```python
from build123d import *

# Parameters (mm, degrees)
SKETCH2_R           = 4.5
BOSS_EXTRUDE1_DEPTH = 17
SKETCH3_R           = 9
BOSS_EXTRUDE2_DEPTH = 18
SKETCH4_R           = 8
BOSS_EXTRUDE3_DEPTH = 29
SKETCH5_R           = 9
BOSS_EXTRUDE4_DEPTH = 15
SKETCH6_R           = 3
BOSS_EXTRUDE5_DEPTH = 20
BOSS_EXTRUDE6_DEPTH = 4
SKETCH17_R          = 3
BOSS_EXTRUDE7_DEPTH = 5
SKETCH18_R          = 9
BOSS_EXTRUDE8_DEPTH = 16
CUT_EXTRUDE1_DEPTH  = 3


with BuildPart() as part:
    # Sketch2 → Boss-Extrude1 (new body)
    with BuildSketch(Plane.YZ):
        Circle(SKETCH2_R)
    extrude(amount=BOSS_EXTRUDE1_DEPTH)

    # Sketch3 → Boss-Extrude2 (add)
    with BuildSketch(Plane(origin=(0, 0, 0), x_dir=(0, -1, 0), z_dir=(-1, 0, 0))):
        Circle(SKETCH3_R)
    extrude(amount=BOSS_EXTRUDE2_DEPTH)

    # Sketch4 → Boss-Extrude3 (add)
    with BuildSketch(Plane(origin=(-18, 0, 0), x_dir=(0, -1, 0), z_dir=(-1, 0, 0))):
        Circle(SKETCH4_R)
    extrude(amount=BOSS_EXTRUDE3_DEPTH)

    # Sketch5 → Boss-Extrude4 (add)
    with BuildSketch(Plane(origin=(-47, 0, 0), x_dir=(0, -1, 0), z_dir=(-1, 0, 0))):
        with Locations((0, -0.197923741)):
            Circle(SKETCH5_R)
    extrude(amount=BOSS_EXTRUDE4_DEPTH)

    # Sketch6 → Boss-Extrude5 (add)
    with BuildSketch(Plane(origin=(-62, 0, 0), x_dir=(0, -1, 0), z_dir=(-1, 0, 0))):
        Circle(SKETCH6_R)
    extrude(amount=BOSS_EXTRUDE5_DEPTH)

    # Sketch16 → Boss-Extrude6 (add, symmetric)
    with BuildSketch(Plane(origin=(0, 0, 0), x_dir=(0, 1, 0), z_dir=(0, 0, 1))):
        with BuildLine():
            Line((0, 62), (-20, 62))
            ThreePointArc((-20, 62), (-34.142135624, 67.857864376), (-40, 82))
            Line((-40, 82), (-40, 102))
            ThreePointArc((-40, 102), (-34.142135624, 116.142135624), (-20, 122))
            Line((-20, 122), (0, 122))
            Line((0, 122), (0, 138))
            Line((0, 138), (-12, 138))
            Line((-12, 138), (-28.922313782, 140.983860496))
            ThreePointArc((-28.922313782, 140.983860496), (-57.497566339, 133.327144649), (-70, 106.51558914))
            Line((-70, 106.51558914), (-70, 82))
            ThreePointArc((-70, 82), (-59.748737342, 57.251262658), (-35, 47))
            Line((-35, 47), (0, 47))
            Line((0, 47), (0, 62))
        make_face()
    extrude(amount=BOSS_EXTRUDE6_DEPTH, both=True)



with BuildPart() as body_2:
    # Sketch17 → Boss-Extrude7 (new body)
    with BuildSketch(Plane.ZY.offset(117)):
        Circle(SKETCH17_R)
    extrude(amount=BOSS_EXTRUDE7_DEPTH)


with BuildPart() as part_1:
    add(part.part)

    add(body_2.part)  # Boss-Extrude8 merges body 2
    # Sketch18 → Boss-Extrude8 (add)
    with BuildSketch(Plane(origin=(-122, 0, 0), x_dir=(0, -1, 0), z_dir=(-1, 0, 0))):
        Circle(SKETCH18_R)
    extrude(amount=BOSS_EXTRUDE8_DEPTH)

    # Sketch21 → Cut-Extrude1 (cut)
    with BuildSketch(Plane.XY.offset(4)):
        with BuildLine():
            Line((-106.51558914, -65), (-82, -65))
            ThreePointArc((-82, -65), (-60.786796564, -56.213203436), (-52, -35))
            Line((-52, -35), (-52, -24.70089464))
            ThreePointArc((-52, -24.70089464), (-54.470885592, -22.009811643), (-57.362613993, -24.24254767))
            ThreePointArc((-57.362613993, -24.24254767), (-65.891984786, -39.11888715), (-82, -45))
            Line((-82, -45), (-102, -45))
            ThreePointArc((-102, -45), (-117.587304364, -39.545739757), (-126.373231569, -25.562875413))
            ThreePointArc((-126.373231569, -25.562875413), (-130.955140822, -22.001423997), (-135.353853676, -25.786810875))
            Line((-135.353853676, -25.786810875), (-136.059821731, -29.79055467))
            ThreePointArc((-136.059821731, -29.79055467), (-129.496922434, -54.283628291), (-106.51558914, -65))
        make_face()
    cut_extrude1 = extrude(amount=-CUT_EXTRUDE1_DEPTH, mode=Mode.SUBTRACT)

    # Mirror1: Cut-Extrude1 across plane
    add(cut_extrude1.mirror(Plane.XY), mode=Mode.SUBTRACT)


solid = part_1.part
```
Input: part model. Units: mm. Frame: model coordinates. A direction names the side the tool comes from. Give positions to 0.01 mm unless a question says otherwise; leave off trailing zeros. Order: outer loops, then holes, each group sorted by start corner. A loop starts at its lowest first (then second) coordinate and runs counter-clockwise, first axis right, second up. Notation, with made-up numbers: (85, -18) - (99, -18) arc R28 cw to (99, 4) - close; hole circle Ø6 at (15, 76.5). An arc over 180 degrees is marked (long way). Put each result on its own line as item: value.
Item 1: Section query D-D, the plane y = -17.5. Return loops of the section in (x, z), then the cut area to 3 significant figures.
Found:
outline: (-138.97, -4) - (-122, -4) - (-122, 4) - (-138.97, 4) - close; (-62, -4) - (-47, -4) - (-47, 4) - (-62, 4) - close
area: 256 mm^2
Item 2: Section query C-C, the plane y = -50. Return loops of the section in (x, z), then the cut area to 3 significant figures.
Found:
outline: (-138.14, -4) - (-132.5, -4) - (-132.5, -1) - (-56.02, -1) - (-56.02, -4) - (-50.38, -4) - (-50.38, 4) - (-56.02, 4) - (-56.02, 1) - (-132.5, 1) - (-132.5, 4) - (-138.14, 4) - close
area: 243 mm^2
Item 3: Access query for faces 1 (the cylindrical face through (-130.9, -22, -2.5)), 2 (the cylindrical face through (-54.4, 9, -0.1)), 3 (the flat face through (-98, -41, 4)). Directions: +Z, -Z, +X, -X, +Y, -Y. A direction counts if a zero-diameter tool reaches every point of the face in a straight line with its end or side. Return the directions, or none.
Found:
face 1: -Z
face 2: none
face 3: +Z, +X, -X, -Y
Item 4: Draft query along X for faces 4 (the cylindrical face through (-8.874, 1.172, 8.923)), 5 (the cylindrical face through (-57.525, -60.019, 0.056)), 6 (the cylindrical face through (-119, 0, -3)). Return one class per face: +X half, -X half, draft (parallel to the pull), parting line (faces both ways), or undercut.
Found:
face 4: draft
face 5: +X half
face 6: undercut
Item 5: Section query A-A, the plane y = 0. Return loops of the section in (x, z).
Found:
outline: (-138, -9) - (-122, -9) - (-122, -3) - (-117, -3) - (-117, 3) - (-122, 3) - (-122, 9) - (-138, 9) - close; (-82, -3) - (-62, -3) - (-62, -9.2) - (-47, -9.2) - (-47, -8) - (-18, -8) - (-18, -9) - (0, -9) - (0, -4.5) - (17, -4.5) - (17, 4.5) - (0, 4.5) - (0, 9) - (-18, 9) - (-18, 8) - (-47, 8) - (-47, 8.8) - (-62, 8.8) - (-62, 3) - (-82, 3) - close
Item 6: Ray query, L1, parallel to Y at x = -70.5, z = -1.75; L2, parallel to X at y = 3, z = -3.5; L3, parallel to X at y = -43, z = 2. Return the intervals inside material, ascending. Write a range as from..to.
Found:
L1: y = -68.06..-62.71, -42.2..-36.36, -2.44..2.44
L2: x = -138..-122, -62..0
L3: x = -140.59..-135.43, -111.8..-72.2, -53.09..-47.93
Item 7: Section query B-B, the plane x = -128.5. Return loops of the section in (y, z).
Found:
outline: (-62.23, -4) - (-55.41, -4) - (-55.41, -1) - (-22.64, -1) - (-22.64, -4) - (-8.06, -4) arc R9 ccw (long way) to (-8.06, 4) - (-22.64, 4) - (-22.64, 1) - (-55.41, 1) - (-55.41, 4) - (-62.23, 4) - close
Item 8: Contact query for flat-ended pins moving along their axis: pin 1 (10 mm diameter, centred on y = -6, z = 3, fed in from -X); pin 2 (1.5 mm diameter, centred on x = -90.5, z = -3, fed in from +Y); pin 3 (3.5 mm diameter, centred on y = -29.5, z = -2, fed in from -X); pin 4 (4 mm diameter, centred on x = -68, y = -6.5, fed in from +Z). Output: stop coordinate, or through.
Found:
pin 1: stops at x = -138
pin 2: stops at y = -40
pin 3: stops at x = -141.31
pin 4: passes through
